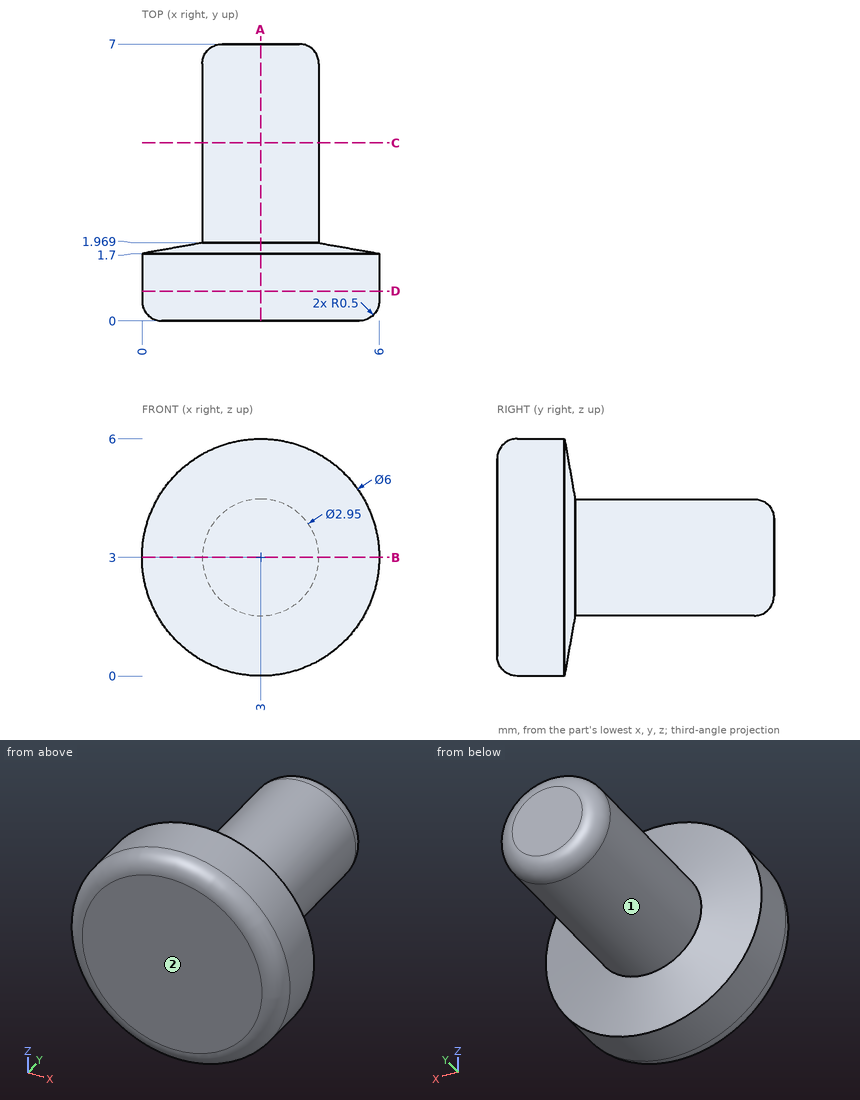
Design review of the part shown in the three views and the two pictorial views. Dimensions are in mm from the part's minimum x, y and z. A direction names the side the tool comes from. Coordinates: 2 decimals unless noted, no trailing zeros. Order: outer loops, then holes, each group sorted by start corner. A loop starts at its lowest first (then second) coordinate and runs counter-clockwise, first axis right, second up. Notation, with made-up numbers: (64.25, 54.5) - (68.25, 54.5) arc R27 cw to (68.25, 79.5) - close; hole circle Ø2 at (68.25, 4). An arc over 180 degrees is marked (long way). One line per question, with ' | ' between items.
Q1. Consider section D-D, the plane y = 0.75. Give the boundary of the cut face in (x, z).
Answer key:
outline: circle Ø6 at (3, 3)
Q2. For the marked faces 1 and 2, list the 3-axis set-ups (+Z, -Z, +X, -X, +Y, -Y) from which the entire face can be reached by the end or side of a thin tool; tool diameter is ignored.
Answer key:
face 1: +Y | face 2: +Z, -Z, +X, -X, -Y
Q3. Consider section C-C, the plane y = 4.5. Give the boundary of the cut face in (x, z) (3 decimals).
Answer key:
outline: circle Ø2.95 at (3, 3)
Q4. Consider section A-A, the plane x = 3. Give the boundary of the cut face in (y, z) (3 decimals).
Answer key:
outline: (0, 0.5) arc R0.5 ccw to (0.5, 0) - (1.7, 0) - (1.969, 1.525) - (6.5, 1.525) arc R0.5 ccw to (7, 2.025) - (7, 3.975) arc R0.5 ccw to (6.5, 4.475) - (1.969, 4.475) - (1.7, 6) - (0.5, 6) arc R0.5 ccw to (0, 5.5) - close
Q5. Clearance check with a flat-ended pin moving along its axis: pin 1 Ø1 at (x, y) = (3.5, 5) entering from -Z (3 decimals). State where the tip first meets the part, or that it passes through.
Answer key:
pin 1: stops at z = 1.525
Q6. To check wall thickness, follow line 1 along X through (y, z) = (5.5, 2.95); line 2 along Y through (x, z) = (2.3, 3.85); line 3 along Y through (x, z) = (2.75, 4.65) (1 decimal). State the ranges of each line that lie inside material, in increasing order.
Answer key:
line 1: x = 1.53 to 4.47 | line 2: y = 0 to 6.98 | line 3: y = 0 to 1.9
Q7. Consider section B-B, the plane z = 3. Give the boundary of the cut face in (x, y) (3 decimals).
Answer key:
outline: (0, 0.5) arc R0.5 ccw to (0.5, 0) - (5.5, 0) arc R0.5 ccw to (6, 0.5) - (6, 1.7) - (4.475, 1.969) - (4.475, 6.5) arc R0.5 ccw to (3.975, 7) - (2.025, 7) arc R0.5 ccw to (1.525, 6.5) - (1.525, 1.969) - (0, 1.7) - close
